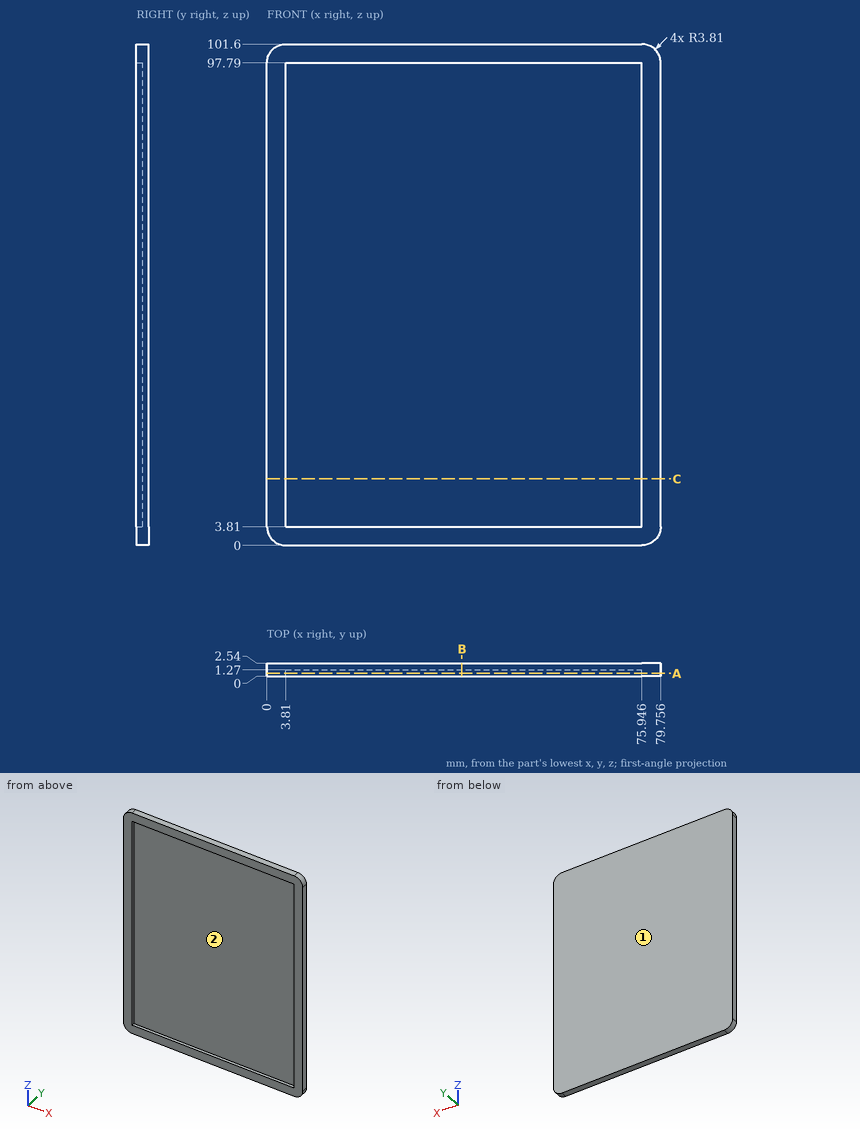
Here's the drawing with two shaded views (mm, measured from the low corner). I have some questions. Coordinates: 2 decimals unless noted, no trailing zeros. Loops run counter-clockwise (first coordinate to the right, second up) from the corner with the lowest first, then second, coordinate; pieces in that order, holes last. Notation, with made-up numbers: (45.5, -27) - (97.5, -27) arc R18 ccw to (97.5, -19) - close; hole circle Ø5 at (2.25, 75.5). An arc over 180 degrees is marked (long way). Answer as CSV lines item,"result". Start each with the question number.
1) Suppose I cut it at C-C (z = 13.5). Please give me the cut outline in (x, y), plus the area to 3 significant figures.
2) I need wall thicknesses on line 1 (Z direction, x = 19, y = 0.9); line 2 (X direction, y = 0.25, z = 11.5); line 3 (Y direction, x = 45, z = 63). Which ranges of each line are inside material? Lowest first, please. Write a range as from..to.
3) Thinking about a two-plate mould opening in Z: for the marked faces 1 and 2, which applies, pulls with the +Z half, pulls with the -Z half, needs draft (parallel to the pull), parting line crosses it, or undercut?
4) Suppose I cut it at B-B (x = 39.5). Please give me the cut outline in (y, z).
5) Suppose I cut it at A-A (y = 0.55). Please give me the cut outline in (x, z), plus the area to 3 significant figures.
Check result:
1,outline,"(0, 0) - (3.81, 0) - (3.81, 1.27) - (75.95, 1.27) - (75.95, 0) - (79.76, 0) - (79.76, 2.54) - (0, 2.54) - close"
1,area,"111 mm²"
2,line 1,"z = 0..3.81, 97.79..101.6"
2,line 2,"x = 0..3.81, 75.95..79.76"
2,line 3,"y = 1.27..2.54"
3,face 1,"needs draft"
3,face 2,"undercut"
4,outline,"(0, 0) - (2.54, 0) - (2.54, 101.6) - (0, 101.6) - (0, 97.79) - (1.27, 97.79) - (1.27, 3.81) - (0, 3.81) - close"
5,outline,"(0, 3.81) arc R3.81 ccw to (3.81, 0) - (75.95, 0) arc R3.81 ccw to (79.76, 3.81) - (79.76, 97.79) arc R3.81 ccw to (75.95, 101.6) - (3.81, 101.6) arc R3.81 ccw to (0, 97.79) - close; hole (3.81, 3.81) - (75.95, 3.81) - (75.95, 97.79) - (3.81, 97.79) - close"
5,area,"1,310 mm²"
